Could you check a few things on this model? Use its own coordinates, in mm. A direction names the side the tool comes from. Coordinates: 2 decimals unless noted, no trailing zeros. Loops run counter-clockwise (first coordinate to the right, second up) from the corner with the lowest first, then second, coordinate; pieces in that order, holes last. Notation, with made-up numbers: M -39,25 L -16,25 A12 cw -16,37 Z; hole C -23,13.25 d5. An arc over 180 degrees is marked long. Write each question's results on one line, items separated by ' | '.
```python
from build123d import *

# Parameters (mm, degrees)
CROQUIS1_R              = 4.56
SALIENTE_EXTRUIR4_DEPTH = 1.5
CROQUIS4_R              = 3.25
SALIENTE_EXTRUIR5_DEPTH = 3
CROQUIS5_R              = 5.25
SALIENTE_EXTRUIR6_DEPTH = 3
CROQUIS6_W              = 2.5
CROQUIS6_H              = 1.700541123
SALIENTE_EXTRUIR7_DEPTH = 90


with BuildPart() as part:
    # Croquis1 → Saliente-Extruir4 (new body)
    with BuildSketch(Plane.XY):
        Circle(CROQUIS1_R)
    extrude(amount=SALIENTE_EXTRUIR4_DEPTH)

    # Croquis4 → Saliente-Extruir5 (add)
    with BuildSketch(Plane(origin=(0, 0, 0), x_dir=(-1, 0, 0), z_dir=(0, 0, -1))):
        Circle(CROQUIS4_R)
    extrude(amount=SALIENTE_EXTRUIR5_DEPTH)

    # Croquis5 → Saliente-Extruir6 (add)
    with BuildSketch(Plane(origin=(0, 0, -3), x_dir=(-1, 0, 0), z_dir=(0, 0, -1))):
        Circle(CROQUIS5_R)
    extrude(amount=SALIENTE_EXTRUIR6_DEPTH)

    # Croquis6 → Saliente-Extruir7 (add)
    with BuildSketch(Plane(origin=(0, 0, -6), x_dir=(-1, 0, 0), z_dir=(0, 0, -1))):
        Polygon((0, -2.40164141), (0, -1.088943), (-4.096121931, -1.088943), (-4.096121931, -2.40164141), (-2.5, -2.40164141), align=None)
        Polygon((4.096121931, -1.088943), (0, -1.088943), (0, -2.40164141), (2.5, -2.40164141), (4.096121931, -2.40164141), align=None)
        with Locations((1.25, -3.251911972)):
            Rectangle(CROQUIS6_W, CROQUIS6_H)
        with Locations((-1.25, -3.251911972)):
            Rectangle(CROQUIS6_W, CROQUIS6_H)
    extrude(amount=SALIENTE_EXTRUIR7_DEPTH)


solid = part.part
```
(1) Will these pins go through, and if not, where does the flat tip stop? P1, Ø4, axis at x = 0.5, z = -40.5, coming from the -Y side; P2, Ø0.9, axis at y = -3.5, z = -41.5, coming from the +X side; P3, Ø3, axis at x = -1, y = 1.5, coming from the -Z side.
Reported:
P1: stops at y = -4.1 | P2: stops at x = 2.5 | P3: stops at z = -6
(2) Imagine slicing it at C-C, the plane y = 0. List the corners of the cut face in (x, z) for me, and give its area (3 significant figures).
Reported:
outline: M -5.25,-6 L 5.25,-6 L 5.25,-3 L 3.25,-3 L 3.25,0 L 4.56,0 L 4.56,1.5 L -4.56,1.5 L -4.56,0 L -3.25,0 L -3.25,-3 L -5.25,-3 Z | area: 64.7 mm2
(3) If we mould it in two halves opening along Z, with no side actions, what happens to faces 5 (the flat face through (0, 0, 1.5)), 6 (the cylindrical face through (-3.6, -2.8, 0.7)), 7 (the cylindrical face through (2.579, -1.978, -1.479))? For each: released by +Z, released by -Z, zero draft, split by the parting line, or undercut.
Reported:
face 5: released by +Z | face 6: zero draft | face 7: undercut
(4) Please list where these lines run through material, in increasing order: probe 1 along Z at (x, y) = (0.5, 3.5); probe 2 along Z at (x, y) = (3, -2.25); probe 3 along Z at (x, y) = (-2.5, -4.25). Write a range as from..to.
Reported:
probe 1: z = -6..-3, 0..1.5 | probe 2: z = -96..-3, 0..1.5 | probe 3: z = -6..-3
(5) Which directions (+Z, -Z, +X, -X, +Y, -Y) give clear straight access to the entire face, cutting with the end or side of a thin tool? Please do faces 1 (the flat face through (0, -1.089, -50)), 2 (the flat face through (0.1, -3.4, -3)), 3 (the flat face through (-2.5, -3, -50)), 4 (the flat face through (2.5, -3, -50)).
Reported:
face 1: -Z, +X, -X, +Y | face 2: none | face 3: -Z, -X, -Y | face 4: -Z, +X, -Y
(6) Imagine slicing it at A-A, the plane x = 0. List the corners of the cut face in (y, z) for me.
Reported:
outline: M -5.25,-6 L -4.1,-6 L -4.1,-96 L -1.09,-96 L -1.09,-6 L 5.25,-6 L 5.25,-3 L 3.25,-3 L 3.25,0 L 4.56,0 L 4.56,1.5 L -4.56,1.5 L -4.56,0 L -3.25,0 L -3.25,-3 L -5.25,-3 Z
(7) Imagine slicing it at B-B, the plane z = -16.5. List the corners of the cut face in (x, y) for me.
Reported:
outline: M -4.1,-2.4 L -2.5,-2.4 L -2.5,-4.1 L 2.5,-4.1 L 2.5,-2.4 L 4.1,-2.4 L 4.1,-1.09 L -4.1,-1.09 Z
